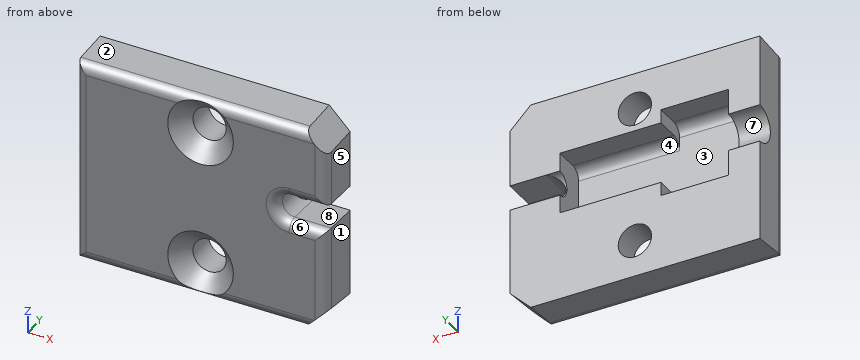
```python
from build123d import *

# Parameters (mm, degrees)
BOSS_EXTRUDE1_DEPTH                             = 3.2
SKETCH2_W                                       = 24
SKETCH2_H                                       = 16.5
BOSS_EXTRUDE2_DEPTH                             = 1
BOSS_EXTRUDE3_DEPTH                             = 4.8
BOSS_EXTRUDE4_DEPTH                             = 3
CUT_EXTRUDE1_REACH                              = 28.659
BOSS_EXTRUDE5_DEPTH                             = 24
SKETCH7_R                                       = 1.55
CUT_EXTRUDE2_DEPTH                              = 10
CHAMFER1_SIZE                                   = 2
FILLET1_R                                       = 1
CSK_FOR_M3_FLAT_HEAD_MACHINE_SCREW1_D           = 3.2
CSK_FOR_M3_FLAT_HEAD_MACHINE_SCREW1_CSINK_D     = 6.3
CSK_FOR_M3_FLAT_HEAD_MACHINE_SCREW1_CSINK_ANGLE = 90
FILLET2_R                                       = 1


with BuildPart() as part:
    # Sketch1 → Boss-Extrude1 (new body)
    with BuildSketch(Plane(origin=(0, 0, 0), x_dir=(1, 0, 0), z_dir=(0, 1, 0))):
        Polygon((1, 8.25), (1, 1.8), (4, 1.8), (4, 4.25), (10.5, 4.25), (10.5, 2.95), (20.2, 2.95), (20.2, 1.2), (25, 1.2), (25, 8.25), align=None)
    extrude(amount=BOSS_EXTRUDE1_DEPTH)


with BuildPart() as body_2:
    # Mirror3: mirrored copy
    add(part.part.mirror(Plane.XY))


with BuildPart() as part_1:
    add(part.part)

    add(body_2.part)  # Boss-Extrude2 merges body 2
    # Sketch2 → Boss-Extrude2 (add)
    with BuildSketch(Plane.XZ):
        with Locations((13, 0)):
            Rectangle(SKETCH2_W, SKETCH2_H)
    extrude(amount=BOSS_EXTRUDE2_DEPTH)

    # Sketch4 → Boss-Extrude3 (add)
    with BuildSketch(Plane(origin=(25, 0, 0), x_dir=(0, 0, -1), z_dir=(1, 0, 0))):
        with BuildLine():
            Line((-1.2, 3.2), (-1.2, 0))
            Line((-1.2, 0), (1.2, 0))
            Line((1.2, 0), (1.2, 3.2))
            ThreePointArc((1.2, 3.2), (0, 2), (-1.2, 3.2))
        make_face()
    extrude(amount=-BOSS_EXTRUDE3_DEPTH)

    # Sketch5 → Boss-Extrude4 (add)
    with BuildSketch(Plane.ZY.offset(-1)):
        with BuildLine():
            Line((-1.8, 3.2), (-1.8, 0))
            Line((-1.8, 0), (1.8, 0))
            Line((1.8, 0), (1.8, 3.2))
            ThreePointArc((1.8, 3.2), (0, 1.4), (-1.8, 3.2))
        make_face()
    extrude(amount=-BOSS_EXTRUDE4_DEPTH)

    # Cut-Extrude1: up to this face of the body (flat: up to its plane)
    cut_extrude1_end = Plane(part_1.part.faces().sort_by_distance((13.712117152, 3.2, 5.4174866))[0])
    # Sketch6 → Cut-Extrude1 (cut, up to the picked face)
    with BuildSketch(Plane.XZ.offset(1), mode=Mode.PRIVATE) as cut_extrude1_sk1:
        with BuildLine():
            Line((21.5, 1.2), (25, 1.2))
            Line((25, 1.2), (25, -1.2))
            Line((25, -1.2), (21.5, -1.2))
            ThreePointArc((21.5, -1.2), (20.3, 0), (21.5, 1.2))
        make_face()
    cut_extrude1_tool1 = split(extrude(cut_extrude1_sk1.sketch, amount=-CUT_EXTRUDE1_REACH, mode=Mode.PRIVATE), bisect_by=cut_extrude1_end, keep=Keep.BOTH, mode=Mode.PRIVATE)
    add(cut_extrude1_tool1.solids().sort_by(Axis((22.770687, -1, 0), (0, 1, 0)))[0], mode=Mode.SUBTRACT)

    # Sketch8 → Boss-Extrude5 (add)
    with BuildSketch(Plane(origin=(25, 0, 0), x_dir=(0, 0, -1), z_dir=(1, 0, 0))):
        Polygon((-8.25, 3.2), (-8.605155295, 3.2), (-8.25, -1), align=None)
        Polygon((8.25, 3.2), (8.25, -1), (11.07, -1), (11.452307692, 3.2), align=None)
    extrude(amount=-BOSS_EXTRUDE5_DEPTH)

    # Sketch7 → Cut-Extrude2 (cut)
    with BuildSketch(Plane(origin=(0, 3.2, 0), x_dir=(1, 0, 0), z_dir=(0, 1, 0))):
        with Locations(Location((13, 7.952307692, 0), (0, 0, 270))):
            Circle(SKETCH7_R)
        with Locations(Location((13, -5.105155295, 0), (0, 0, 90))):
            Circle(SKETCH7_R)
    extrude(amount=-CUT_EXTRUDE2_DEPTH, mode=Mode.SUBTRACT)

    # Chamfer1
    chamfer1_edges = [part_1.edges().sort_by_distance(p)[0] for p in [
        (25, 1.1, 8.427577647),
        (25, 1.1, -11.261153846),
    ]]
    chamfer(chamfer1_edges, length=CHAMFER1_SIZE)

    # Fillet1
    fillet1_edges = [part_1.edges().sort_by_distance(p)[0] for p in [
        (25, -1, 3.721431105),
        (20.3, -1, 0),
        (23.25, -1, -1.2),
        (23.25, -1, 1.2),
        (12, -1, -11.07),
        (12, -1, 8.25),
        (25, -1, -5.130865713),
        (1, -1, -1.41),
    ]]
    fillet(fillet1_edges, radius=FILLET1_R)

    # CSK for M3 Flat Head Machine Screw1 (through all)
    with Locations(Plane(origin=(0, -1, 0), x_dir=(-1, 0, 0), z_dir=(0, -1, 0))):
        with Locations((-13, -5.105155295), (-13, 7.952307692)):
            CounterSinkHole(CSK_FOR_M3_FLAT_HEAD_MACHINE_SCREW1_D / 2, CSK_FOR_M3_FLAT_HEAD_MACHINE_SCREW1_CSINK_D / 2, counter_sink_angle=CSK_FOR_M3_FLAT_HEAD_MACHINE_SCREW1_CSINK_ANGLE)

    # Fillet2
    fillet2_edges = [part_1.edges().sort_by_distance(p)[0] for p in [
        (15.35, 0, -2.95),
        (7.25, 0, -4.25),
        (15.35, 0, 2.95),
        (7.25, 0, 4.25),
    ]]
    fillet(fillet2_edges, radius=FILLET2_R)


solid = part_1.part
```
For this review, take the finished solid that the model builds, in its own axes (mm). Face numbers are marked on the shaded views. A direction names the side the tool comes from. Give positions to 0.01 mm unless a question says otherwise; leave off trailing zeros. Loops run counter-clockwise (first coordinate to the right, second up) from the corner with the lowest first, then second, coordinate; pieces in that order, holes last. Notation, with made-up numbers: M 59.5,53 L 93.5,53 A26 cw 93.5,69 Z; hole C 53.5,12.5 d2. An arc over 180 degrees is marked long. One line per item, written item: value. Start each with the question number.
Q1. For L1, parallel to X at y = 1.7, z = 3.25; L2, parallel to Z at x = 13, y = 1.55; L3, parallel to Y at x = 10.5, z = 0, list the stretches that pass through material, from the lowest coordinate up.
Q2. Draft analysis for pull direction X (two halves, no side actions). For the marked faces 1, 2 and 3, state which applies: released by +X, released by -X, zero draft, split by the parting line, or undercut.
Q3. Add section A-A (z = 0). Give the boundary of the cut face in (x, y).
Q4. Add section C-C (x = 13). Give the boundary of the cut face in (y, z).
Q5. Clearance check with flat-ended pins moving along their axes: pin 1 Ø2.5 at (x, y) = (23.5, 1.5) entering from +Z; pin 2 Ø1.1 at (x, y) = (7, 2.5) entering from -Z; pin 3 Ø1.9 at (x, z) = (13, 5.11) entering from -Y; pin 4 Ø1.8 at (x, y) = (15, 1.5) entering from +Z. State where each tip first meets the part, or that it passes through.
Q6. Add section B-B (x = 22.25). Give the boundary of the cut face in (y, z).
Q7. Machinability: for the marked faces 4, 5, 6, 7 and 8, which of the approach directions +Z, -Z, +X, -X, +Y, -Y give a long, thin tool a straight path to every point of the face, cutting with its end or side? Answer none if there is none.
Q8. Add section D-D (y = 1.7). Give the boundary of the cut face in (x, z), and give its area (3 significant figures).
Reply:
1. L1: 1 to 4, 10.5 to 25
1. L2: -11.3 to -9.55, -6.35 to -2.95, 2.95 to 3.51, 6.71 to 8.47
1. L3: -1 to 0
2. face 1: released by +X
2. face 2: zero draft
2. face 3: undercut
3. outline: M 1,0 A1 ccw 2,-1 L 19.3,-1 A1 ccw 20.3,0 L 20.3,2 L 20.2,2 L 20.2,0 L 4,0 L 4,1.4 L 1,1.4 Z
4. outline: M -1,-4.8 L 0.55,-6.35 L 3.2,-6.35 L 3.2,-2.95 L 1,-2.95 A1 cw 0,-1.95 L 0,1.95 A1 cw 1,2.95 L 3.2,2.95 L 3.2,3.51 L 0.55,3.51 L -1,1.96 Z; M -0.74,8 L 0.55,6.71 L 3.2,6.71 L 3.2,8.61 L -0.08,8.33 A1 ccw Z; M -0.73,-10.84 A1 ccw -0.09,-11.15 L 3.2,-11.45 L 3.2,-9.55 L 0.55,-9.55 Z
5. pin 1: z = 8.56
5. pin 2: z = -11.44
5. pin 3: through
5. pin 4: z = 8.54
6. outline: M -1,-10.16 A1 ccw -0.09,-11.15 L 3.2,-11.45 L 3.2,-1.2 L 0,-1.2 A1 ccw -1,-2.2 Z; M -1,2.2 A1 ccw 0,1.2 L 3.2,1.2 L 3.2,8.61 L -0.08,8.33 A1 ccw -1,7.33 Z
7. face 4: +Y
7. face 5: +Z, -Z, +X, +Y, -Y
7. face 6: +X, -Y
7. face 7: -X, +Y
7. face 8: +X, +Y, -Y
8. outline: M 1,-11.32 L 23,-11.32 L 25,-9.31 L 25,-1.2 L 21.5,-1.2 A1.2 cw 21.5,1.2 L 25,1.2 L 25,6.47 L 23,8.48 L 1,8.48 L 1,0.99 L 4,0.99 L 4,4.25 L 10.5,4.25 L 10.5,2.95 L 20.2,2.95 L 20.2,-2.95 L 10.5,-2.95 L 10.5,-4.25 L 4,-4.25 L 4,-0.99 L 1,-0.99 Z; hole C 13,-7.95 d3.2; hole C 13,5.11 d3.2
8. area: 326 mm²
